Can you work these out from the model? Positions are in its coordinate system, mm. A direction names the side the tool comes from. Round coordinates to 2 decimals unless told otherwise and drop trailing zeros. Loops run counter-clockwise (first coordinate to the right, second up) from the corner with the lowest first, then second, coordinate; pieces in that order, holes last. Notation, with made-up numbers: (81, -33) -> (88, -33) arc R17 ccw to (88, -24) -> close; hole circle Ø9 at (28, 2.25). An arc over 180 degrees is marked (long way). Use a Markdown table: item, result.
from build123d import *

# Parameters (mm, degrees)
SKETCH1_R           = 13.5
BOSS_EXTRUDE1_DEPTH = 23
SKETCH2_R           = 12.5
BOSS_EXTRUDE2_DEPTH = 0.1
SKETCH3_R           = 13.5
BOSS_EXTRUDE3_DEPTH = 4
SKETCH4_R           = 12
BOSS_EXTRUDE4_DEPTH = 30
SKETCH5_R           = 11.5
SKETCH5_R_2         = 3
CUT_EXTRUDE1_DEPTH  = 2
SKETCH6_R           = 2.25
SKETCH6_R_2         = 0.5
BOSS_EXTRUDE5_DEPTH = 6
SKETCH7_R           = 2.25
SKETCH7_R_2         = 0.5
BOSS_EXTRUDE6_DEPTH = 20
BOSS_EXTRUDE7_DEPTH = 5
SKETCH9_W           = 0.5
SKETCH9_H           = 0.5
CUT_EXTRUDE2_DEPTH  = 0.5


with BuildPart() as part:
    # Sketch1 → Boss-Extrude1 (new body)
    with BuildSketch(Plane.XY):
        Circle(SKETCH1_R)
    extrude(amount=BOSS_EXTRUDE1_DEPTH)

    # Sketch2 → Boss-Extrude2 (add)
    with BuildSketch(Plane.XY.offset(23)):
        Circle(SKETCH2_R)
    extrude(amount=BOSS_EXTRUDE2_DEPTH)

    # Sketch3 → Boss-Extrude3 (add)
    with BuildSketch(Plane.XY.offset(23.1)):
        Circle(SKETCH3_R)
    extrude(amount=BOSS_EXTRUDE3_DEPTH)

    # Sketch4 → Boss-Extrude4 (add)
    with BuildSketch(Plane(origin=(0, 0, 0), x_dir=(-1, 0, 0), z_dir=(0, 0, -1))):
        Circle(SKETCH4_R)
    extrude(amount=BOSS_EXTRUDE4_DEPTH)

    # Sketch5 → Cut-Extrude1 (cut)
    with BuildSketch(Plane(origin=(0, 0, -30), x_dir=(-1, 0, 0), z_dir=(0, 0, -1))):
        Circle(SKETCH5_R)
        Circle(SKETCH5_R_2, mode=Mode.SUBTRACT)
    extrude(amount=-CUT_EXTRUDE1_DEPTH, mode=Mode.SUBTRACT)

    # Sketch6 → Boss-Extrude5 (add)
    with BuildSketch(Plane.XY.offset(27.1)):
        Circle(SKETCH6_R)
        Circle(SKETCH6_R_2, mode=Mode.SUBTRACT)
    extrude(amount=BOSS_EXTRUDE5_DEPTH)

    # Sketch7 → Boss-Extrude6 (add)
    with BuildSketch(Plane(origin=(0, 0, 0), x_dir=(1, 0, 0), z_dir=(0, 1, 0))):
        with Locations(Location((0, -5, 0), (0, 0, 90))):
            Circle(SKETCH7_R)
        with Locations(Location((0, -5, 0), (0, 0, 90))):
            Circle(SKETCH7_R_2, mode=Mode.SUBTRACT)
    extrude(amount=BOSS_EXTRUDE6_DEPTH)

    # Sketch8 → Boss-Extrude7 (add)
    with BuildSketch(Plane(origin=(0, 0, -28), x_dir=(-1, 0, 0), z_dir=(0, 0, -1))):
        Polygon((0.549485189, 5.995670607), (1.2440779, 9.934901619), (2.228885653, 9.761253441), (1.534292943, 5.822022429), align=None)
        Polygon((-2.228885653, -9.761253441), (-1.2440779, -9.934901619), (-0.549485189, -5.995670607), (-1.534292943, -5.822022429), align=None)
    extrude(amount=BOSS_EXTRUDE7_DEPTH)

    # Sketch9 → Cut-Extrude2 (cut)
    with BuildSketch(Plane(origin=(0, 0, -30), x_dir=(-1, 0, 0), z_dir=(0, 0, -1))):
        Rectangle(SKETCH9_W, SKETCH9_H)
    extrude(amount=-CUT_EXTRUDE2_DEPTH, mode=Mode.SUBTRACT)


solid = part.part
1. I want a section at C-C (z = -9). Please give me the cut outline in (x, y), plus the area to 3 significant figures.
Answer sheet:
| item | result |
|---|---|
| outline | circle Ø24 at (0, 0) |
| area | 452 mm² |
2. I want a section at D-D (y = 8). Please give me the cut outline in (x, z), plus the area to 3 significant figures.
Answer sheet:
| item | result |
|---|---|
| outline | (-10.87, 0) -> (-8.94, 0) -> (-8.94, -30) -> (-8.26, -30) -> (-8.26, -28) -> (-1.92, -28) -> (-1.92, -33) -> (-0.9, -33) -> (-0.9, -28) -> (8.26, -28) -> (8.26, -30) -> (8.94, -30) -> (8.94, 0) -> (10.87, 0) -> (10.87, 23) -> (9.6, 23) -> (9.6, 23.1) -> (10.87, 23.1) -> (10.87, 27.1) -> (-10.87, 27.1) -> (-10.87, 23.1) -> (-9.6, 23.1) -> (-9.6, 23) -> (-10.87, 23) -> close |
| area | 1,100 mm² |
3. I need wall thicknesses on line 1 (Y direction, x = 0, z = -28.8); line 2 (X direction, y = 16.5, z = 5); line 3 (Z direction, x = -5.75, y = 1). Which ranges of each line are inside material? Lowest first, please.
Answer sheet:
| item | result |
|---|---|
| line 1 | y = -12 to -11.5, -3 to 3, 11.5 to 12 |
| line 2 | x = -2.25 to -0.5, 0.5 to 2.25 |
| line 3 | z = -28 to 27.1 |
4. Which directions (+Z, -Z, +X, -X, +Y, -Y) give clear straight access to the entire face, cutting with the end or side of a thin tool? Please do faces 1 (the flat face through (-1.4, 7.9, -33)), 2 (the cylindrical face through (-0.676, 16.609, 2.854)), 3 (the cylindrical face through (3, 0, -29)).
Answer sheet:
| item | result |
|---|---|
| face 1 | -Z, +X, -X, +Y, -Y |
| face 2 | +Y |
| face 3 | -Z |
5. If we mould it in two halves opening along Y, with no side actions, what happens to faces 4 (the flat face through (-2.4, -2.4, -28)), 5 (the flat face through (-1, 20, 5)), 6 (the flat face through (-1, 0, -30))? For each: +Y half, -Y half, draft (parallel to the pull), parting line (faces both ways), or undercut.
Answer sheet:
| item | result |
|---|---|
| face 4 | undercut |
| face 5 | +Y half |
| face 6 | draft |
6. I want a section at A-A (x = 7.25). Please give me the cut outline in (y, z), plus the area to 3 significant figures.
Answer sheet:
| item | result |
|---|---|
| outline | (-11.39, 0) -> (-9.56, 0) -> (-9.56, -30) -> (-8.93, -30) -> (-8.93, -28) -> (8.93, -28) -> (8.93, -30) -> (9.56, -30) -> (9.56, 0) -> (11.39, 0) -> (11.39, 23) -> (10.18, 23) -> (10.18, 23.1) -> (11.39, 23.1) -> (11.39, 27.1) -> (-11.39, 27.1) -> (-11.39, 23.1) -> (-10.18, 23.1) -> (-10.18, 23) -> (-11.39, 23) -> close |
| area | 1,160 mm² |
7. I want a section at B-B (y = 16). Please give me the cut outline in (x, z), plus the area to 3 significant figures.
Answer sheet:
| item | result |
|---|---|
| outline | circle Ø4.5 at (0, 5); hole circle Ø1 at (0, 5) |
| area | 15.1 mm² |
8. Will these pins go through, and if not, where does the flat tip stop? pin 1 Ø2 at (x, y) = (-5, -7.5) entering from +Z; pin 2 Ø7 at (x, y) = (-4, 2.5) entering from -Z; pin 3 Ø4 at (x, y) = (7, -5.5) entering from -Z; pin 4 Ø1.1 at (x, y) = (0, 0) entering from +Z.
Answer sheet:
| item | result |
|---|---|
| pin 1 | stops at z = 27.1 |
| pin 2 | stops at z = -30 |
| pin 3 | stops at z = -28 |
| pin 4 | stops at z = 33.1 |
